Design review of the part shown in the three views and the two pictorial views. Dimensions are in mm from the part's minimum x, y and z. A direction names the side the tool comes from. Round coordinates to 2 decimals unless told otherwise and drop trailing zeros. Order: outer loops, then holes, each group sorted by start corner. A loop starts at its lowest first (then second) coordinate and runs counter-clockwise, first axis right, second up. Notation, with made-up numbers: (16.5, -29) - (66.5, -29) arc R14 cw to (66.5, -24) - close; hole circle Ø3 at (55.5, -13.5). An arc over 180 degrees is marked (long way). Use CSV: the item, a comma, the result in double quotes.
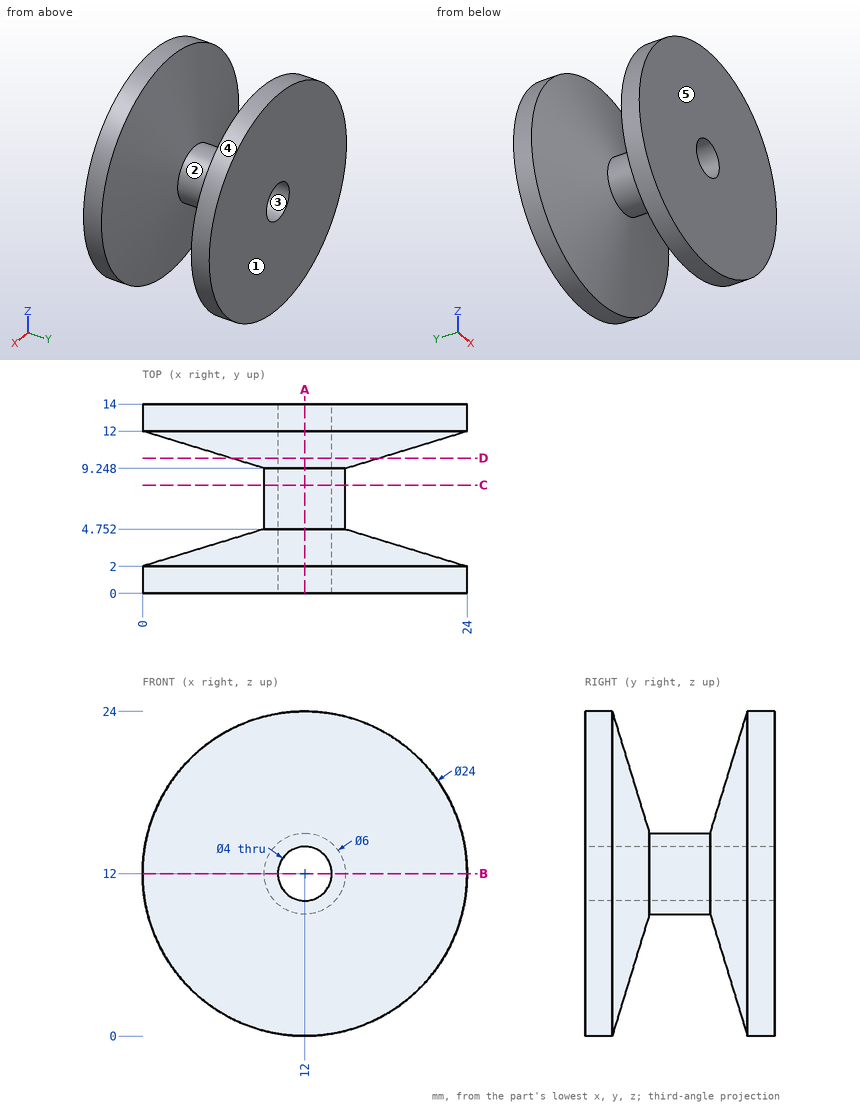
1) We need section B-B (z = 12). Give the boundary of the cut face in (x, y).
Data:
outline,"(0, 0) - (10, 0) - (10, 14) - (0, 14) - (0, 12) - (9, 9.25) - (9, 4.75) - (0, 2) - close; (14, 0) - (24, 0) - (24, 2) - (15, 4.75) - (15, 9.25) - (24, 12) - (24, 14) - (14, 14) - close"
2) We need section A-A (x = 12). Give the boundary of the cut face in (y, z).
Data:
outline,"(0, 0) - (2, 0) - (4.75, 9) - (9.25, 9) - (12, 0) - (14, 0) - (14, 10) - (0, 10) - close; (0, 14) - (14, 14) - (14, 24) - (12, 24) - (9.25, 15) - (4.75, 15) - (2, 24) - (0, 24) - close"
3) We need section D-D (y = 10). Give the boundary of the cut face in (x, z).
Data:
outline,"circle Ø10.92 at (12, 12); hole circle Ø4 at (12, 12)"
4) We need section C-C (y = 8). Give the boundary of the cut face in (x, z).
Data:
outline,"circle Ø6 at (12, 12); hole circle Ø4 at (12, 12)"
5) The part is to be moulded in two halves that separate along Z. For the marked faces 3, 4 and 5, say which applies: +Z half, -Z half, draft (parallel to the pull), parting line (faces both ways), or undercut.
Data:
face 3,"undercut"
face 4,"parting line"
face 5,"draft"
6) For the marked faces 1 and 2, list the 3-axis set-ups (+Z, -Z, +X, -X, +Y, -Y) from which the entire face can be reached by the end or side of a thin tool; tool diameter is ignored.
Data:
face 1,"+Z, -Z, +X, -X, +Y"
face 2,"none"
7) To check wall thickness, follow L1, parallel to Y at x = 14.5, z = 20; L2, parallel to Y at x = 8.25, z = 13.5 (1 decimal); L3, parallel to X at y = 5, z = 10.5 (1 decimal). State the ranges of each line that lie inside material, in increasing order. Write a range as from..to.
Data:
L1,"y = 0..3.11, 10.89..14"
L2,"y = 0..4.4, 9.6..14"
L3,"x = 9.4..10.7, 13.3..14.6"
8) Insertion check: pin 1 Ø1 at (y, z) = (5.5, 16) entering from +X; pin 2 Ø3 at (x, y) = (19, 11) entering from +Z. Each pin has a flat end and moves straight along its axis. Give the tip position at first contact, or say it passes through.
Data:
pin 1,"passes through"
pin 2,"stops at z = 22.46"
